The drawing under review shows one solid part. Ordinate dimensions are in mm from its lowest x, y, z. A direction names the side the tool comes from. Coordinates: 2 decimals unless noted, no trailing zeros. Write each loop counter-clockwise with the first axis right and the second up, starting at its lowest first coordinate (ties: lowest second). Pieces come first, ordered by that corner, then holes. Notation, with made-up numbers: (38.5, -22) - (92.5, -22) arc R30 cw to (92.5, 1) - close; hole circle Ø2 at (-20.75, 13.5). An arc over 180 degrees is marked (long way). Use a Markdown table: item, result.
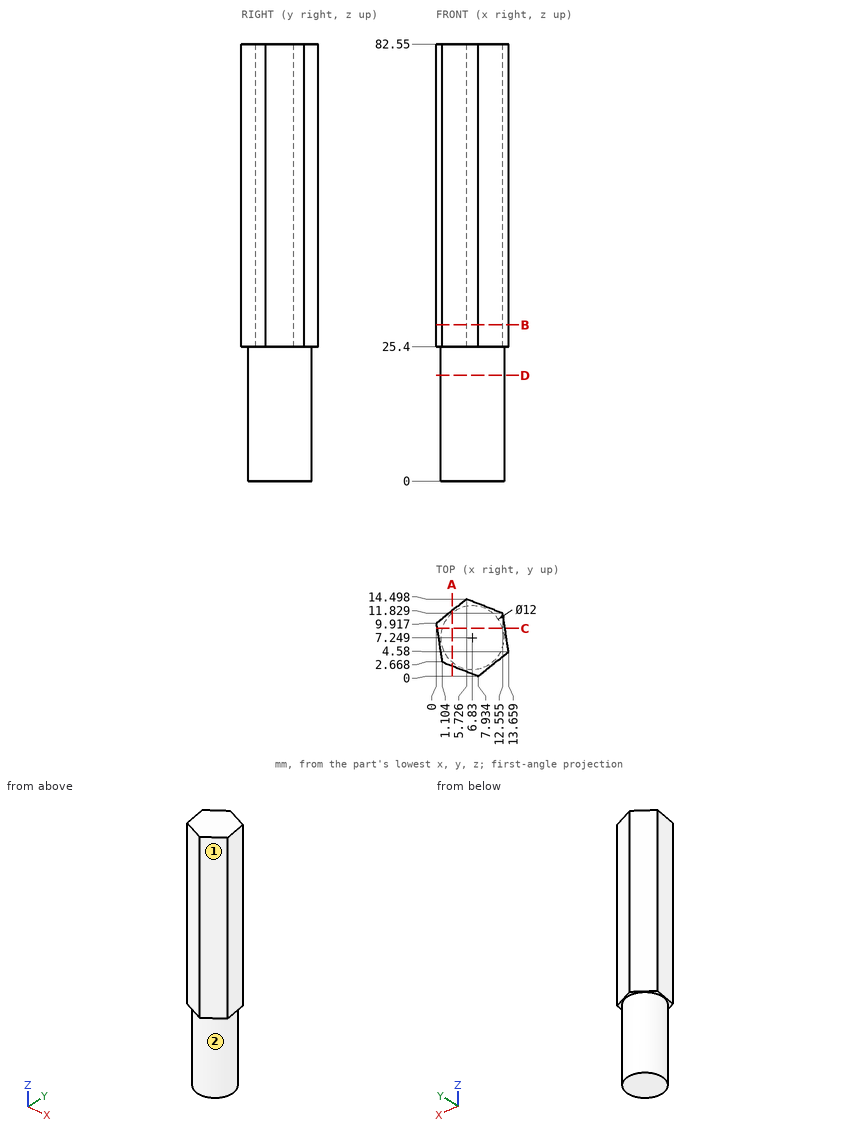
(1) Take a section at D-D on z = 20. Write out the cut boundary in (x, y), and give its area (3 significant figures).
Determined:
| item | result |
|---|---|
| outline | circle Ø12 at (6.83, 7.25) |
| area | 113 mm2 |
(2) Take a section at A-A on x = 3. Write out the cut boundary in (y, z).
Determined:
| item | result |
|---|---|
| outline | (1.93, 25.4) - (2.63, 25.4) - (2.63, 0) - (11.87, 0) - (11.87, 25.4) - (12.32, 25.4) - (12.32, 82.55) - (1.93, 82.55) - close |
(3) Take a section at C-C on y = 9. Write out the cut boundary in (x, z), and give its area (3 significant figures).
Determined:
| item | result |
|---|---|
| outline | (0.14, 25.4) - (1.09, 25.4) - (1.09, 0) - (12.57, 0) - (12.57, 25.4) - (12.99, 25.4) - (12.99, 82.55) - (0.14, 82.55) - close |
| area | 1,030 mm2 |
(4) For pin 1 (4 mm diameter, centred on x = 6, y = 4, fed in from -Z); pin 2 (2 mm diameter, centred on x = 2.5, z = 21, fed in from +Y), all flat-tipped, find the tip position at first contact; note any pin that passes through.
Determined:
| item | result |
|---|---|
| pin 1 | z = 0 |
| pin 2 | y = 12.24 |
(5) For L1, parallel to Z at x = 10, y = 1.75; L2, parallel to Y at x = 3.75, z = 12.5; L3, parallel to Y at x = 7.25, z = 47, list the stretches that pass through material, from the lowest coordinate up. Write a range as from..to.
Determined:
| item | result |
|---|---|
| L1 | 25.4..82.55 |
| L2 | 2.1..12.4 |
| L3 | 0.27..13.9 |
(6) Take a section at B-B on z = 29.5. Write out the cut boundary in (x, y) (1 decimal).
Determined:
| item | result |
|---|---|
| outline | (0, 9.9) - (1.1, 2.7) - (7.9, 0) - (13.7, 4.6) - (12.6, 11.8) - (5.7, 14.5) - close |
(7) Machinability: for the marked faces 1 and 2, which of the approach directions +Z, -Z, +X, -X, +Y, -Y give a long, thin tool a straight path to every point of the face, cutting with its end or side? Answer none if there is none.
Determined:
| item | result |
|---|---|
| face 1 | +Z, -Z, +X, -Y |
| face 2 | -Z |
